```python
from build123d import *

# Parameters (mm, degrees)
BOSS_EXTRUDE1_DEPTH = 4
BOSS_EXTRUDE1_DRAFT = 1
SHELL1_T            = -0.5
SKETCH2_R           = 2
BOSS_EXTRUDE2_DEPTH = 5.5
BOSS_EXTRUDE2_TAPER = 1.5
CIRPATTERN1_COUNT   = 4
SKETCH4_R           = 1.605977431
CUT_EXTRUDE1_DEPTH  = 5.5
CUT_EXTRUDE1_DRAFT  = 1.5
RIB2_START          = -8.069744096
RIB2_DEPTH          = 6.231928651
RIB2_START_2        = 1.837815445
RIB2_2_DEPTH        = 6.231928651
RIB2_START_3        = -5.944744096
RIB2_3_DEPTH        = 4.106928651
RIB2_4_DEPTH        = 4.106928651


with BuildPart() as part:
    # Sketch1 → Boss-Extrude1 (with draft: the straight prism first)
    with BuildSketch(Plane(origin=(0, 0, 0), x_dir=(1, 0, 0), z_dir=(0, 1, 0))):
        with BuildLine():
            Line((-7.5, -6.375), (7.5, -6.375))
            ThreePointArc((7.5, -6.375), (8.207106781, -6.082106781), (8.5, -5.375))
            Line((8.5, -5.375), (8.5, 5.375))
            ThreePointArc((8.5, 5.375), (8.207106781, 6.082106781), (7.5, 6.375))
            Line((7.5, 6.375), (-7.5, 6.375))
            ThreePointArc((-7.5, 6.375), (-8.207106781, 6.082106781), (-8.5, 5.375))
            Line((-8.5, 5.375), (-8.5, -5.375))
            ThreePointArc((-8.5, -5.375), (-8.207106781, -6.082106781), (-7.5, -6.375))
        make_face()
    extrude(amount=-BOSS_EXTRUDE1_DEPTH)
    # Boss-Extrude1: the draft: its side faces are tilted about the plane it starts from
    boss_extrude1_sides = [part.faces().sort_by_distance(p)[0] for p in [
        (0, -2, 6.375),
        (8.207106781, -2, 6.082106781),
        (8.5, -2, 0),
        (8.207106781, -2, -6.082106781),
        (0, -2, -6.375),
        (-8.207106781, -2, -6.082106781),
        (-8.5, -2, 0),
        (-8.207106781, -2, 6.082106781),
    ]]
    draft(boss_extrude1_sides, Plane(origin=(0, 0, 0), x_dir=(1, 0, 0), z_dir=(0, 1, 0)), BOSS_EXTRUDE1_DRAFT)

    # Shell1
    shell1_openings = [part.faces().sort_by_distance(p)[0] for p in [
        (0, -4, 0),
    ]]
    offset(amount=SHELL1_T, openings=shell1_openings, kind=Kind.INTERSECTION)

    # Sketch2 → Boss-Extrude2 (add)
    with BuildSketch(Plane.XZ.offset(0.5)):
        Circle(SKETCH2_R)
    extrude(amount=BOSS_EXTRUDE2_DEPTH, taper=BOSS_EXTRUDE2_TAPER)

    # Rib1: read off the stored shape, not the designer's step
    # Rib1: loft between two sections, ruled curve by curve
    rib1_from = [
        Edge.make_line((-1.982384256, -0.5, 0.264863479), (-2.837165081, -0.5, 0.25)),
        Edge.make_line((-2.837165081, -0.5, -0.25), (-1.982384256, -0.5, -0.264863479)),
        Edge.make_line((-2.837165081, -0.5, -0.25), (-2.837165081, -0.5, 0.25)),
        Edge.make_line((-1.982384256, -0.5, -0.264863479), (-1.982384256, -0.5, 0.264863479)),
    ]
    rib1_to = [
        Edge.make_line((-1.837815545, -6, 0.259010132), (-2.355977431, -6, 0.25)),
        Edge.make_line((-2.355977431, -6, -0.25), (-1.837815545, -6, -0.259010132)),
        Edge.make_line((-2.355977431, -6, -0.25), (-2.355977431, -6, 0.25)),
        Edge.make_line((-1.837815545, -6, -0.259010132), (-1.837815545, -6, 0.259010132)),
    ]
    rib1 = Solid(Shell([*[Face.make_surface_from_curves(rib1_from[k], rib1_to[k]) for k in range(4)], Face(Wire(rib1_from)), Face(Wire(rib1_to))]))
    add(rib1)

    # CirPattern1: Rib1 ×4 about axis
    cirpattern1_axis = Axis((0, 0, 0), (0, 1, 0))
    for i in range(1, CIRPATTERN1_COUNT):
        add(rib1.rotate(cirpattern1_axis, i * 360 / CIRPATTERN1_COUNT))


with BuildPart() as cut_extrude1_tool:
    # Sketch4 → Cut-Extrude1 (with draft: the straight prism first)
    with BuildSketch(Plane.XZ.offset(6)):
        Circle(SKETCH4_R)
    extrude(amount=-CUT_EXTRUDE1_DEPTH)
    # Cut-Extrude1: the draft: its side faces are tilted about the plane it starts from
    cut_extrude1_sides = [cut_extrude1_tool.faces().sort_by_distance(p)[0] for p in [
        (-1.605977431, -3.25, 0),
    ]]
    draft(cut_extrude1_sides, Plane.XZ.offset(6), CUT_EXTRUDE1_DRAFT)


with BuildPart() as part_1:
    add(part.part)

    # Cut-Extrude1: cut by cut_extrude1_tool
    add(cut_extrude1_tool.part, mode=Mode.SUBTRACT)

    # Sweep1: sweep along a path in Sketch6
    with BuildLine(Plane(origin=(0, -2, 0), x_dir=(1, 0, 0), z_dir=(0, 1, 0))) as sweep1_path:
        Line((-8.56982026, 5.375), (-8.56982026, -5.375))
        ThreePointArc((-8.56982026, -5.375), (-8.25647716, -6.13147716), (-7.5, -6.44482026))
        Line((-7.5, -6.44482026), (7.5, -6.44482026))
        ThreePointArc((7.5, -6.44482026), (8.25647716, -6.13147716), (8.56982026, -5.375))
        Line((8.56982026, -5.375), (8.56982026, 5.375))
        ThreePointArc((8.56982026, 5.375), (8.25647716, 6.13147716), (7.5, 6.44482026))
        Line((7.5, 6.44482026), (-7.5, 6.44482026))
        ThreePointArc((-7.5, 6.44482026), (-8.25647716, 6.13147716), (-8.56982026, 5.375))
    # Sketch5 → Sweep1 (sweep)
    with BuildSketch(Plane(origin=(0, 0, 0), x_dir=(0, 0, -1), z_dir=(1, 0, 0))):
        Polygon((6.44482026, -4), (6.40991013, -2), (6.70991013, -2), align=None)
    sweep(path=sweep1_path.line)

    # Rib2: read off the stored shape, not the designer's step
    # Rib2 outline → Rib2 (add)
    with BuildSketch(Plane.YZ.offset(RIB2_START)):
        Polygon((-2, -0.25), (-0.5, -0.276182597), (-0.5, 0.276182597), (-2, 0.25), align=None)
    extrude(amount=RIB2_DEPTH)

    # Rib2 2 outline → Rib2 2 (add)
    with BuildSketch(Plane.YZ.offset(RIB2_START_2)):
        Polygon((-2, -0.25), (-0.5, -0.276182597), (-0.5, 0.276182597), (-2, 0.25), align=None)
    extrude(amount=RIB2_2_DEPTH)

    # Rib2 3 outline → Rib2 3 (add)
    with BuildSketch(Plane.XY.offset(RIB2_START_3)):
        Polygon((-0.276182597, -0.5), (-0.25, -2), (0.25, -2), (0.276182597, -0.5), align=None)
    extrude(amount=RIB2_3_DEPTH)

    # Rib2 4 outline → Rib2 4 (add)
    with BuildSketch(Plane.XY.offset(RIB2_START_2)):
        Polygon((-0.276182597, -0.5), (-0.25, -2), (0.25, -2), (0.276182597, -0.5), align=None)
    extrude(amount=RIB2_4_DEPTH)


solid = part_1.part
```
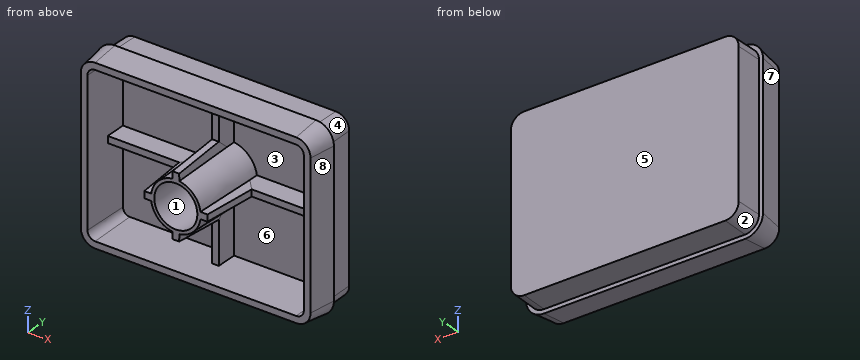
Here's how the part is built. I have some questions about the finished solid (model axes, mm). Face numbers are marked on the shaded views. A direction names the side the tool comes from. Round coordinates to 2 decimals unless told otherwise and drop trailing zeros. Order: outer loops, then holes, each group sorted by start corner. A loop starts at its lowest first (then second) coordinate and runs counter-clockwise, first axis right, second up. Notation, with made-up numbers: (43.25, -5.5) -> (57.25, -5.5) arc R12 cw to (57.25, -1.5) -> close; hole circle Ø3 at (-5, 58). An arc over 180 degrees is marked (long way). Use a Markdown table: item, result. Add a question column.
(1) Suppose I cut it at A-A, the plane x = -4.5. Please give me the cut outline in (y, z) (3 decimals).
(2) If we mould it in two halves opening along X, with no side actions, what happens to the marked faces 5, 6, 7 and 8? For each: released by +X, released by -X, zero draft, split by the parting line, or undercut.
(3) For pin 1 Ø1 at (x, z) = (7, -0.5) entering from +Y; pin 2 Ø0.6 at (x, z) = (5.5, 0) entering from -Y; pin 3 Ø6 at (x, z) = (6, 4) entering from -Y; pin 4 Ø3 at (x, z) = (-5.5, -3.5) entering from -Y, each with a flat end and sliding along its axis, tell me the tip position at first contact or that it passes through.
(4) For the marked faces 1, 2, 3 and 4, which set-ups out of +Z, -Z, +X, -X, +Y, -Y let a thin tool reach every point of the face, with its end or its side?
(5) Suppose I cut it at C-C, the plane y = -2.75. Count the separate pieces of the cut face and the enclosed holes in it, and give its area (3 significant figures).
(6) Suppose I cut it at B-B, the plane z = -4.75. Please give me the cut outline in (x, y), and give its area (3 significant figures).
(7) I need wall thicknesses on line 1 along Z through (x, y) = (0, -2.25); line 2 along Y through (x, z) = (7.75, -5.25); line 3 along X through (y, z) = (-0.75, 4). Which ranges of each line are inside material? Lowest first, please.
Verdict:
| question | item | result |
|---|---|---|
| 1 | outline | (-4, -6.445) -> (-2, -6.71) -> (-2, -6.41) -> (0, -6.375) -> (0, 6.375) -> (-2, 6.41) -> (-2, 6.71) -> (-4, 6.445) -> (-4, 5.945) -> (-0.5, 5.884) -> (-0.5, 0.276) -> (-2, 0.25) -> (-2, -0.25) -> (-0.5, -0.276) -> (-0.5, -5.884) -> (-4, -5.945) -> close |
| 2 | face 5 | zero draft |
| 2 | face 6 | undercut |
| 2 | face 7 | released by -X |
| 2 | face 8 | released by +X |
| 3 | pin 1 | y = 0 |
| 3 | pin 2 | y = -2 |
| 3 | pin 3 | y = -4 |
| 3 | pin 4 | y = -0.5 |
| 4 | face 1 | none |
| 4 | face 2 | -Z, -X, +Y |
| 4 | face 3 | -Y |
| 4 | face 4 | +Z, +X, +Y |
| 5 | separate pieces | 2 |
| 5 | enclosed holes | 2 |
| 5 | area | 43.6 mm2 |
| 6 | outline | (-8.83, -2) -> (-8.57, -4) -> (-8.07, -4) -> (-8.01, -0.5) -> (-0.28, -0.5) -> (-0.25, -2) -> (0.25, -2) -> (0.28, -0.5) -> (8.01, -0.5) -> (8.07, -4) -> (8.57, -4) -> (8.83, -2) -> (8.53, -2) -> (8.5, 0) -> (-8.5, 0) -> (-8.53, -2) -> close |
| 6 | area | 13.4 mm2 |
| 7 | line 1 | -6.68 to -5.91, -2.68 to -1.7, 1.7 to 2.68, 5.91 to 6.68 |
| 7 | line 2 | -0.5 to 0 |
| 7 | line 3 | -8.51 to -8.01, -0.27 to 0.27, 8.01 to 8.51 |
